from build123d import *

# Parameters (mm, degrees)
SKETCH_W          = 20
SKETCH_H          = 20
PAD_DEPTH         = 31
SKETCH001_R       = 2.5
PAD001_DEPTH      = 16
PAD001_DEPTH_BACK = 38.5
SKETCH002_R       = 2.5
PAD002_DEPTH      = 16.3
SKETCH003_W       = 20
SKETCH003_H       = 18
SKETCH003_R       = 8.5
POCKET_DEPTH      = 29
SKETCH004_R       = 1.45
HOLE_DEPTH        = 2
HOLE_TIPS_R       = 1.45
SKETCH005_R       = 5
PAD003_DEPTH      = 6


with BuildPart() as part:
    # Sketch → Pad (new body)
    with BuildSketch(Plane.XZ):
        Rectangle(SKETCH_W, SKETCH_H)
    extrude(amount=-PAD_DEPTH)

    # Sketch001 → Pad001 (join, two sides)
    with BuildSketch(Plane.XZ) as pad001_sk:
        Circle(SKETCH001_R)
    extrude(amount=PAD001_DEPTH)
    extrude(pad001_sk.sketch, amount=-PAD001_DEPTH_BACK)

    # Sketch002 → Pad002 (join)
    with BuildSketch(Plane.XY):
        with Locations((0, -3)):
            Circle(SKETCH002_R)
    extrude(amount=PAD002_DEPTH)

    # Sketch003 → Pocket (cut)
    with BuildSketch(Plane.XZ.offset(-1)):
        Rectangle(SKETCH003_W, SKETCH003_H)
        Circle(SKETCH003_R, mode=Mode.SUBTRACT)
    extrude(amount=-POCKET_DEPTH, mode=Mode.SUBTRACT)

    # Sketch004 → Hole (cut)
    with BuildSketch(Plane.XY.offset(-10)):
        with Locations((-5, 23)):
            Circle(SKETCH004_R)
        with Locations((-5, 8)):
            Circle(SKETCH004_R)
        with Locations((5, 8)):
            Circle(SKETCH004_R)
        with Locations((5, 23)):
            Circle(SKETCH004_R)
    extrude(amount=HOLE_DEPTH, mode=Mode.SUBTRACT)

    # Hole tips → Hole tip 1 section 0
    with BuildSketch(Plane.XY.offset(-8), mode=Mode.PRIVATE) as hole_tip_1_s0:
        with Locations((-5, 23)):
            Circle(HOLE_TIPS_R)
    loft([hole_tip_1_s0.sketch, Vertex(-5, 23, -7.128752)], mode=Mode.SUBTRACT)

    # Hole tips → Hole tip 2 section 0
    with BuildSketch(Plane.XY.offset(-8), mode=Mode.PRIVATE) as hole_tip_2_s0:
        with Locations((-5, 8)):
            Circle(HOLE_TIPS_R)
    loft([hole_tip_2_s0.sketch, Vertex(-5, 8, -7.128752)], mode=Mode.SUBTRACT)

    # Hole tips → Hole tip 3 section 0
    with BuildSketch(Plane.XY.offset(-8), mode=Mode.PRIVATE) as hole_tip_3_s0:
        with Locations((5, 8)):
            Circle(HOLE_TIPS_R)
    loft([hole_tip_3_s0.sketch, Vertex(5, 8, -7.128752)], mode=Mode.SUBTRACT)

    # Hole tips → Hole tip 4 section 0
    with BuildSketch(Plane.XY.offset(-8), mode=Mode.PRIVATE) as hole_tip_4_s0:
        with Locations((5, 23)):
            Circle(HOLE_TIPS_R)
    loft([hole_tip_4_s0.sketch, Vertex(5, 23, -7.128752)], mode=Mode.SUBTRACT)

    # Sketch005 → Pad003 (join)
    with BuildSketch(Plane.XZ):
        Circle(SKETCH005_R)
    extrude(amount=PAD003_DEPTH)


solid = part.part
Geometry check sheet. Reference: the model listing, model coordinates, mm. A direction names the side the tool comes from. Round coordinates to 2 decimals unless told otherwise and drop trailing zeros. Order: outer loops, then holes, each group sorted by start corner. A loop starts at its lowest first (then second) coordinate and runs counter-clockwise, first axis right, second up. Notation, with made-up numbers: M 32,65 L 68,65 A24 cw 68,89 Z; hole C 63.5,76.25 d2. An arc over 180 degrees is marked long. Answer in a Markdown table with one row per item.
(1) Go/stop test with flat-tipped pins: P1, Ø1, axis at x = -2.5, y = -2, coming from the -Z side; P2, Ø2.5, axis at x = -5, y = 23, coming from the -Z side; P3, Ø4, axis at y = 18.5, z = 6, coming from the +X side. Record where each tip stops, or that it passes through.
Responses:
| item | result |
|---|---|
| P1 | stops at z = -4.58 |
| P2 | stops at z = -7.63 |
| P3 | stops at x = 7.5 |
(2) Sectioned sample at B-B, the plane z = 0. Record the cut outline in (x, y), and give its area (4 significant figures).
Responses:
| item | result |
|---|---|
| outline | M -10,0 L -5,0 L -5,-6 L -2.5,-6 L -2.5,-16 L 2.5,-16 L 2.5,-6 L 5,-6 L 5,0 L 10,0 L 10,1 L 8.5,1 L 8.5,30 L 10,30 L 10,31 L 2.5,31 L 2.5,38.5 L -2.5,38.5 L -2.5,31 L -10,31 L -10,30 L -8.5,30 L -8.5,1 L -10,1 Z |
| area | 680.5 mm² |
(3) Sectioned sample at A-A, the plane y = 3. Record the cut outline in (x, z).
Responses:
| item | result |
|---|---|
| outline | M -10,-10 L 10,-10 L 10,-9 L -10,-9 Z; M -10,9 L 10,9 L 10,10 L -10,10 Z; C 0,0 d17 |
(4) Tool access check on faces 5 (the face through (-0.54, 34.7, -2.44)), 6 (the face through (2, -6, -2)), 7 (the face through (2.31, -3.96, 10.23)), 8 (the face through (-2, 0, 5)). Record the directions out of +Z, -Z, +X, -X, +Y, -Y that give a thin tool (end or side, any length) a straight path to the whole face; none if there is none.
Responses:
| item | result |
|---|---|
| face 5 | +Y |
| face 6 | -Y |
| face 7 | +Z |
| face 8 | none |
(5) Draft check along Z on faces 1 (the face through (3.85, 22.12, -9.51)), 2 (the face through (-9, 30, 0)), 3 (the face through (-0.54, -10.93, -2.44)), 4 (the face through (0, 15, 9)). Enter one of: released by +Z, released by -Z, zero draft, split by the parting line, or undercut.
Responses:
| item | result |
|---|---|
| face 1 | zero draft |
| face 2 | undercut |
| face 3 | split by the parting line |
| face 4 | undercut |
(6) Sectioned sample at D-D, the plane y = -11. Record the cut outline in (x, z).
Responses:
| item | result |
|---|---|
| outline | C 0,0 d5 |
(7) Scan lines: probe 1 along X at (y, z) = (23, -9.45); probe 2 along Y at (x, z) = (-5, -9.7); probe 3 along Z at (x, y) = (-9, 29). Record each from-to range of solid material in increasing order. Write a range as from..to.
Responses:
| item | result |
|---|---|
| probe 1 | x = -10..-6.45, -3.55..3.55, 6.45..10 |
| probe 2 | y = 0..6.55, 9.45..21.55, 24.45..31 |
| probe 3 | z = -10..-9, 9..10 |
(8) Sectioned sample at C-C, the plane x = 7.75. Record the cut outline in (y, z).
Responses:
| item | result |
|---|---|
| outline | M 0,-10 L 31,-10 L 31,10 L 0,10 Z; hole M 1,-9 L 30,-9 L 30,-3.49 L 1,-3.49 Z; hole M 1,3.49 L 30,3.49 L 30,9 L 1,9 Z |
